Input: part model. Units: mm. Frame: model coordinates. Round coordinates to 2 decimals unless told otherwise and drop trailing zeros. Order: outer loops, then holes, each group sorted by start corner. A loop starts at its lowest first (then second) coordinate and runs counter-clockwise, first axis right, second up. Notation, with made-up numbers: M 55.25,11.5 L 90.25,11.5 A15 cw 90.25,25.5 Z; hole C -7,83.5 d11. An arc over 180 degrees is marked long. One line per question, with ' | ' between items.
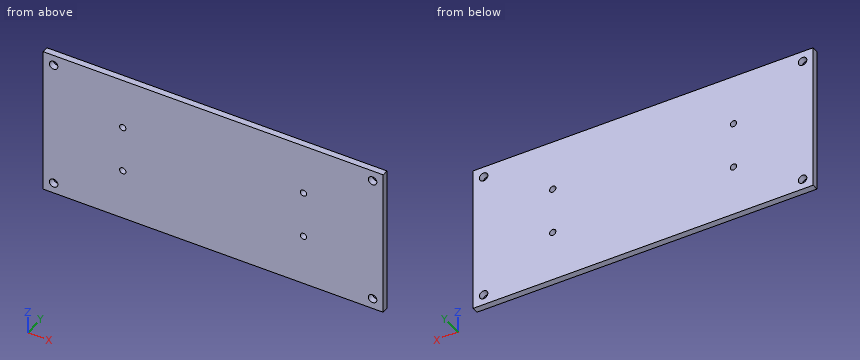
```python
from build123d import *

# Parameters (mm, degrees)
SKETCH1_W      = 160
SKETCH1_H      = 70
EXTRUDE1_DEPTH = 3
SKETCH2_R      = 2
EXTRUDE2_DEPTH = 120
SKETCH3_R      = 1.5
EXTRUDE3_DEPTH = 10


with BuildPart() as part:
    # Sketch1 → Extrude1 (new body)
    with BuildSketch(Plane(origin=(0, 0, 0), x_dir=(1, 0, 0), z_dir=(0, 1, 0))):
        Rectangle(SKETCH1_W, SKETCH1_H)
    extrude(amount=EXTRUDE1_DEPTH)

    # Sketch2 → Extrude2 (cut)
    with BuildSketch(Plane(origin=(0, 3, 0), x_dir=(1, 0, 0), z_dir=(0, 1, 0))):
        with Locations(Location((-75, 30, 0), (0, 0, 270))):
            Circle(SKETCH2_R)
        with Locations(Location((-75, -30, 0), (0, 0, 270))):
            Circle(SKETCH2_R)
        with Locations(Location((75, -30, 0), (0, 0, 270))):
            Circle(SKETCH2_R)
        with Locations(Location((75, 30, 0), (0, 0, 270))):
            Circle(SKETCH2_R)
    extrude(amount=-EXTRUDE2_DEPTH, mode=Mode.SUBTRACT)

    # Sketch3 → Extrude3 (cut)
    with BuildSketch(Plane(origin=(0, 3, 0), x_dir=(1, 0, 0), z_dir=(0, 1, 0))):
        with Locations(Location((-42.5, 11, 0), (0, 0, 270))):
            Circle(SKETCH3_R)
        with Locations(Location((-42.5, -11, 0), (0, 0, 270))):
            Circle(SKETCH3_R)
        with Locations(Location((42.5, -11, 0), (0, 0, 270))):
            Circle(SKETCH3_R)
        with Locations(Location((42.5, 11, 0), (0, 0, 270))):
            Circle(SKETCH3_R)
    extrude(amount=-EXTRUDE3_DEPTH, mode=Mode.SUBTRACT)


solid = part.part
```
Item 1: First-contact query: pin 1 (5 mm diameter, centred on x = 75, z = -30, fed in from -Y); pin 2 (2.5 mm diameter, centred on x = -42.5, z = 11, fed in from -Y). Flat tips, straight axial feed; report the tip coordinate or a pass-through.
Report:
pin 1: y = 0 | pin 2: through
Item 2: Section query B-B, the plane x = -75. Return loops of the section in (y, z).
Report:
outline: M 0,-35 L 3,-35 L 3,-32 L 0,-32 Z; M 0,-28 L 3,-28 L 3,28 L 0,28 Z; M 0,32 L 3,32 L 3,35 L 0,35 Z
Item 3: Section query A-A, the plane z = -30. Return loops of the section in (x, y).
Report:
outline: M -80,0 L -77,0 L -77,3 L -80,3 Z; M -73,0 L 73,0 L 73,3 L -73,3 Z; M 77,0 L 80,0 L 80,3 L 77,3 Z
Item 4: Line query: line 1 along X through (y, z) = (2.05, 11); line 2 along X through (y, z) = (1.5, 30); line 3 along Z through (x, y) = (-74, 1.9). Output: solid intervals per line, ascending. Write a range as from..to.
Report:
line 1: -80..-44, -41..41, 44..80 | line 2: -80..-77, -73..73, 77..80 | line 3: -35..-31.73, -28.27..28.27, 31.73..35
